from build123d import *

# Parameters (mm, degrees)
SKETCH1_W           = 22.4
SKETCH1_H           = 19
BOSS_EXTRUDE1_DEPTH = 3
FILLET2_R           = 1.3
BOSS_EXTRUDE2_REACH = 220.391


with BuildPart() as part:
    # Sketch1 → Boss-Extrude1 (new body)
    with BuildSketch(Plane(origin=(0, 0, 0), x_dir=(1, 0, 0), z_dir=(0, 1, 0))):
        Polygon((-1.892946275, -20.564259839), (226.707053725, -20.564259839), (226.707053725, -17.564259839), (215.507053725, -17.564259839), (215.507053725, 1.435740161), (226.707053725, 1.435740161), (226.707053725, 4.435740161), (-1.892946275, 4.435740161), (-1.892946275, 1.435740161), (9.307053725, 1.435740161), (9.307053725, -17.564259839), (-1.892946275, -17.564259839), align=None)
        with Locations((23.507053725, -8.064259839)):
            Rectangle(SKETCH1_W, SKETCH1_H, mode=Mode.SUBTRACT)
        with Locations((201.307053725, -8.064259839)):
            Rectangle(SKETCH1_W, SKETCH1_H, mode=Mode.SUBTRACT)
        with Locations((175.907053725, -8.064259839)):
            Rectangle(SKETCH1_W, SKETCH1_H, mode=Mode.SUBTRACT)
        with Locations((150.507053725, -8.064259839)):
            Rectangle(SKETCH1_W, SKETCH1_H, mode=Mode.SUBTRACT)
        with Locations((125.107053725, -8.064259839)):
            Rectangle(SKETCH1_W, SKETCH1_H, mode=Mode.SUBTRACT)
        with Locations((99.707053725, -8.064259839)):
            Rectangle(SKETCH1_W, SKETCH1_H, mode=Mode.SUBTRACT)
        with Locations((74.307053725, -8.064259839)):
            Rectangle(SKETCH1_W, SKETCH1_H, mode=Mode.SUBTRACT)
        with Locations((48.907053725, -8.064259839)):
            Rectangle(SKETCH1_W, SKETCH1_H, mode=Mode.SUBTRACT)
    extrude(amount=BOSS_EXTRUDE1_DEPTH)

    # Fillet2
    fillet2_edges = [part.edges().sort_by_distance(p)[0] for p in [
        (113.907053725, 0, 8.064259839),
        (125.107053725, 0, 17.564259839),
        (110.907053725, 0, 8.064259839),
        (125.107053725, 0, -1.435740161),
        (139.307053725, 0, 8.064259839),
        (150.507053725, 0, 17.564259839),
        (3.707053725, 0, -1.435740161),
        (136.307053725, 0, 8.064259839),
        (150.507053725, 0, -1.435740161),
        (9.307053725, 0, 8.064259839),
        (161.707053725, 0, 8.064259839),
        (3.707053725, 0, 17.564259839),
        (175.907053725, 0, -1.435740161),
        (164.707053725, 0, 8.064259839),
        (175.907053725, 0, 17.564259839),
        (-1.892946275, 0, 19.064259839),
        (187.107053725, 0, 8.064259839),
        (112.407053725, 0, 20.564259839),
        (201.307053725, 0, -1.435740161),
        (190.107053725, 0, 8.064259839),
        (201.307053725, 0, 17.564259839),
        (212.507053725, 0, 8.064259839),
        (226.707053725, 0, -2.935740161),
        (221.107053725, 0, -1.435740161),
        (215.507053725, 0, 8.064259839),
        (221.107053725, 0, 17.564259839),
        (23.507053725, 0, 17.564259839),
        (226.707053725, 0, 19.064259839),
        (12.307053725, 0, 8.064259839),
        (23.507053725, 0, -1.435740161),
        (112.407053725, 0, -4.435740161),
        (-1.892946275, 0, -2.935740161),
        (34.707053725, 0, 8.064259839),
        (48.907053725, 0, -1.435740161),
        (37.707053725, 0, 8.064259839),
        (48.907053725, 0, 17.564259839),
        (60.107053725, 0, 8.064259839),
        (74.307053725, 0, -1.435740161),
        (63.107053725, 0, 8.064259839),
        (74.307053725, 0, 17.564259839),
        (85.507053725, 0, 8.064259839),
        (99.707053725, 0, -1.435740161),
        (88.507053725, 0, 8.064259839),
        (99.707053725, 0, 17.564259839),
    ]]
    fillet(fillet2_edges, radius=FILLET2_R)

    # Boss-Extrude2: up to this face of the body (flat: up to its plane)
    boss_extrude2_end = Plane(part.part.faces().sort_by_distance((9.307053725, 2.15, 8.064259839))[0])
    # Sketch2 → Boss-Extrude2 (add, up to the picked face)
    with BuildSketch(Plane(origin=(215.507053725, 0, 0), x_dir=(0, 0, -1), z_dir=(1, 0, 0)), mode=Mode.PRIVATE) as boss_extrude2_sk1:
        with BuildLine():
            Line((2.935740161, 1.3), (1.43659757, 1.3))
            Line((1.43659757, 1.3), (1.43659757, -0.960067332))
            ThreePointArc((1.43659757, -0.960067332), (1.588401468, -1.617613734), (2.013087264, -2.142069327))
            Line((2.013087264, -2.142069327), (5.035485323, -4.503499992))
            Line((5.035485323, -4.503499992), (8.250046613, -1.991930219))
            ThreePointArc((8.250046613, -1.991930219), (8.533170477, -1.642293157), (8.634373075, -1.203928889))
            Line((8.634373075, -1.203928889), (8.634373075, 3))
            Line((8.634373075, 3), (7.098760361, 3))
            Line((7.098760361, 3), (7.098760361, -0.691652004))
            Line((7.098760361, -0.691652004), (6.098760361, -1.691652004))
            Line((6.098760361, -1.691652004), (3.935740161, -1.691652004))
            Line((3.935740161, -1.691652004), (2.935740161, -0.691652004))
            Line((2.935740161, -0.691652004), (2.935740161, 1.3))
        make_face()
    boss_extrude2_tool1 = split(extrude(boss_extrude2_sk1.sketch, amount=-BOSS_EXTRUDE2_REACH, mode=Mode.PRIVATE), bisect_by=boss_extrude2_end, keep=Keep.BOTH, mode=Mode.PRIVATE)
    add(boss_extrude2_tool1.solids().sort_by(Axis((215.507054, 1.196024, -2.186169), (-1, 0, 0)))[0])


solid = part.part
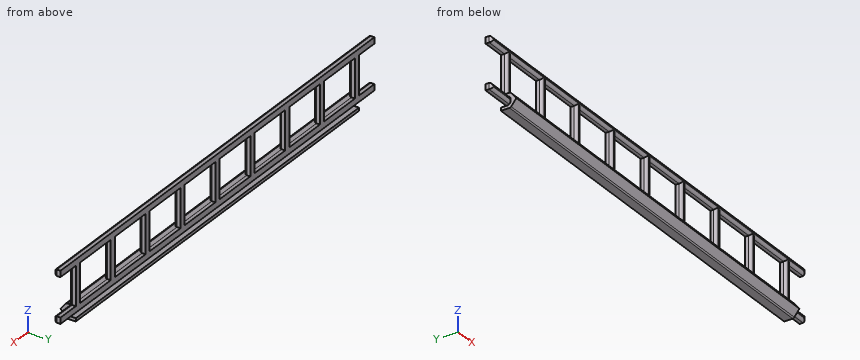
Design review of the part built by this model. Coordinates are the model's own, in mm. Give positions to 0.01 mm unless a question says otherwise; leave off trailing zeros. Write each loop counter-clockwise with the first axis right and the second up, starting at its lowest first coordinate (ties: lowest second). Pieces come first, ordered by that corner, then holes. Notation, with made-up numbers: M 46.25,34 L 53.25,34 A21 ccw 53.25,40 Z; hole C 78.5,-24 d10. An arc over 180 degrees is marked long. Answer as a JSON object with one key per item and string values. Group by question number.
1) For line 1 along Z through (x, y) = (193, 0.75); line 2 along Z through (x, y) = (206, -0.5); line 3 along X through (y, z) = (-2.5, -5.75), list the stretches that pass through material, from the lowest coordinate up.
2) We need section B-B (z = 8). Count the separate pieces of the cut face and the enclosed holes in it, and give its area (3 significant figures).
3) We need section A-A (x = 73.5). Give the boundary of the cut face in (y, z).
4) Clearance check with flat-ended pins moving along their axes: pin 1 Ø0.5 at (y, z) = (2.5, 7.5) entering from -X; pin 2 Ø0.8 at (y, z) = (2.5, 10.5) entering from +X; pin 3 Ø1.4 at (x, y) = (3, 2.5) entering from -Z. State where each tip first meets the part, or that it passes through.
Answer key:
{
 "1": {"line 1": "z = -8.63 to -7.1, -4.31 to -1.44, 17.69 to 20.44", "line 2": "z = -8.63 to -7.1, -2.94 to -1.44", "line 3": "x = 9.31 to 215.51"},
 "2": {"separate pieces": "9", "enclosed holes": "0", "area": "74.5 mm²"},
 "3": {"outline": "M -4.5,-5.04 L -1.99,-8.25 A1 ccw -1.2,-8.63 L 3,-8.63 L 3,-7.1 L -0.69,-7.1 L -1.69,-6.1 L -1.69,-3.94 L -0.69,-2.94 L 0,-2.94 L 0,-3.14 A1.3 ccw 1.3,-4.44 L 3,-4.44 L 3,-1.44 L 1.3,-1.44 A1.3 ccw 1.25,-1.44 L -0.96,-1.44 A1.5 ccw -2.14,-2.01 Z; M 0,18.86 A1.3 ccw 1.3,17.56 L 3,17.56 L 3,20.56 L 1.3,20.56 A1.3 ccw 0,19.26 Z"},
 "4": {"pin 1": "stops at x = 9.31", "pin 2": "stops at x = 215.51", "pin 3": "stops at z = -4.44"}
}
